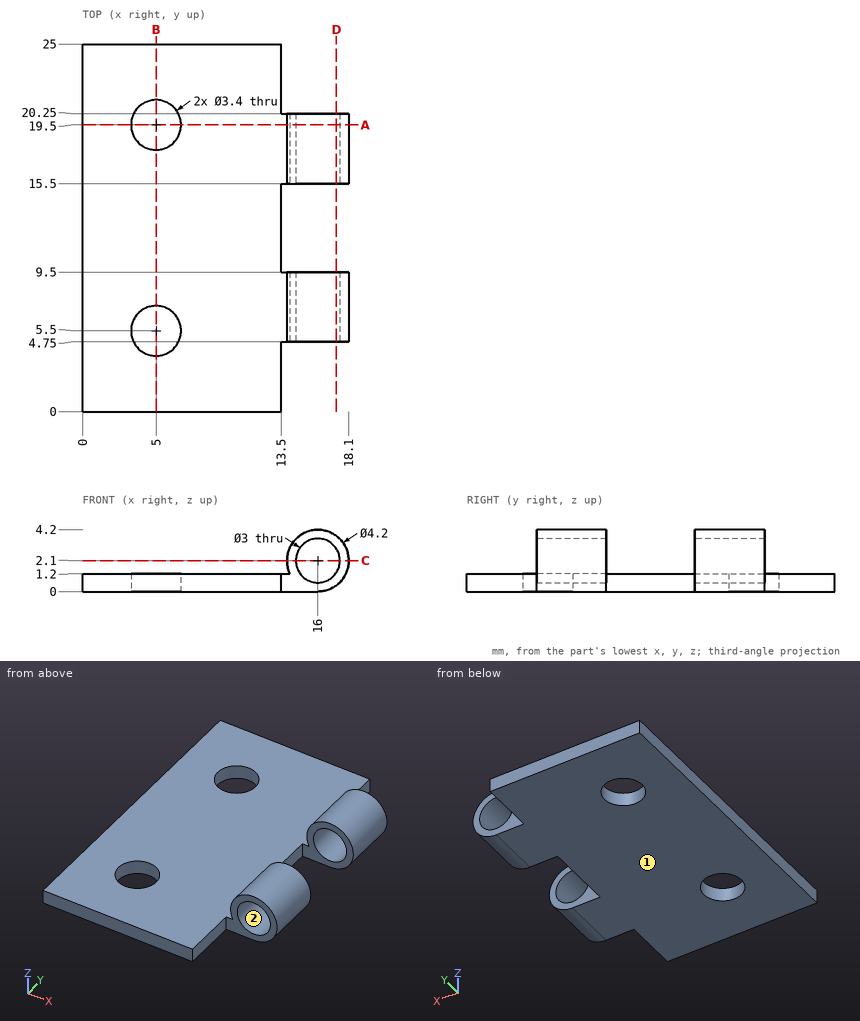
Drawing for the job (mm, zero at the part's lowest x, y, z). Coordinates: 2 decimals unless noted, no trailing zeros. Write each loop counter-clockwise with the first axis right and the second up, starting at its lowest first coordinate (ties: lowest second). Pieces come first, ordered by that corner, then holes. Notation, with made-up numbers: (77.5, -20.5) -> (112.5, -20.5) arc R17 ccw to (112.5, -7.5) -> close; hole circle Ø3 at (49.5, -7). An arc over 180 degrees is marked (long way). One line per item, written item: value. Start each with the question number.
1) Pull direction Z, two halves, no side cores. Call the marked faces 1 and 2: +Z half, -Z half, draft (parallel to the pull), parting line (faces both ways), or undercut.
2) Slice it at A-A on y = 19.5. Write the cut outline in (x, z), then the cut area to 3 significant figures.
3) Slice it at B-B on x = 5. Write the cut outline in (y, z).
4) Flat gauge pins, fed straight in: pin 1 Ø3 at (x, y) = (3, 15) entering from +Z; pin 2 Ø1.5 at (x, z) = (14.5, 2.5) entering from -Y; pin 3 Ø1 at (y, z) = (22, 0.5) entering from +X; pin 4 Ø5.5 at (x, y) = (5, 5.5) entering from -Z. Where does each tip first touch, or does it go through?
5) Slice it at D-D on x = 17.25. Write the cut outline in (y, z).
6) Probe probe 1 along Y at (x, z) = (5, 0.55); probe 2 along X at (y, z) = (5.75, 2.1); probe 3 along Z at (x, y) = (6, 3). List the from-to ranges inside material, lowest first.
7) Slice it at C-C on z = 2.1. Write the cut outline in (x, y), then the cut area to 3 significant figures.
Answers follow:
1. face 1: -Z half
1. face 2: undercut
2. outline: (0, 0) -> (3.3, 0) -> (3.3, 1.2) -> (0, 1.2) -> close; (6.7, 0) -> (16, 0) arc R2.1 ccw (long way) to (14.1, 1.2) -> (6.7, 1.2) -> close; hole circle Ø3 at (16, 2.1)
2. area: 20.3 mm2
3. outline: (0, 0) -> (3.8, 0) -> (3.8, 1.2) -> (0, 1.2) -> close; (7.2, 0) -> (17.8, 0) -> (17.8, 1.2) -> (7.2, 1.2) -> close; (21.2, 0) -> (25, 0) -> (25, 1.2) -> (21.2, 1.2) -> close
4. pin 1: z = 1.2
4. pin 2: y = 4.75
4. pin 3: x = 13.5
4. pin 4: z = 0
5. outline: (4.75, 0.41) -> (9.5, 0.41) -> (9.5, 1.27) -> (4.75, 1.27) -> close; (4.75, 2.93) -> (9.5, 2.93) -> (9.5, 3.79) -> (4.75, 3.79) -> close; (15.5, 0.41) -> (20.25, 0.41) -> (20.25, 1.27) -> (15.5, 1.27) -> close; (15.5, 2.93) -> (20.25, 2.93) -> (20.25, 3.79) -> (15.5, 3.79) -> close
6. probe 1: 0 to 3.8, 7.2 to 17.8, 21.2 to 25
6. probe 2: 13.9 to 14.5, 17.5 to 18.1
6. probe 3: 0 to 1.2
7. outline: (13.9, 4.75) -> (14.5, 4.75) -> (14.5, 9.5) -> (13.9, 9.5) -> close; (13.9, 15.5) -> (14.5, 15.5) -> (14.5, 20.25) -> (13.9, 20.25) -> close; (17.5, 4.75) -> (18.1, 4.75) -> (18.1, 9.5) -> (17.5, 9.5) -> close; (17.5, 15.5) -> (18.1, 15.5) -> (18.1, 20.25) -> (17.5, 20.25) -> close
7. area: 11.4 mm2
